Geometry check sheet. Reference: drawing and pictorial views, mm from the part's lowest x, y, z. Give positions to 0.01 mm unless a question says otherwise; leave off trailing zeros. Write each loop counter-clockwise with the first axis right and the second up, starting at its lowest first coordinate (ties: lowest second). Pieces come first, ordered by that corner, then holes. Notation, with made-up numbers: M 47.25,41.5 L 100.25,41.5 A28 cw 100.25,71.5 Z; hole C 2.25,29 d3. An arc over 180 degrees is marked long. Answer as a JSON object with one key per item and string values.
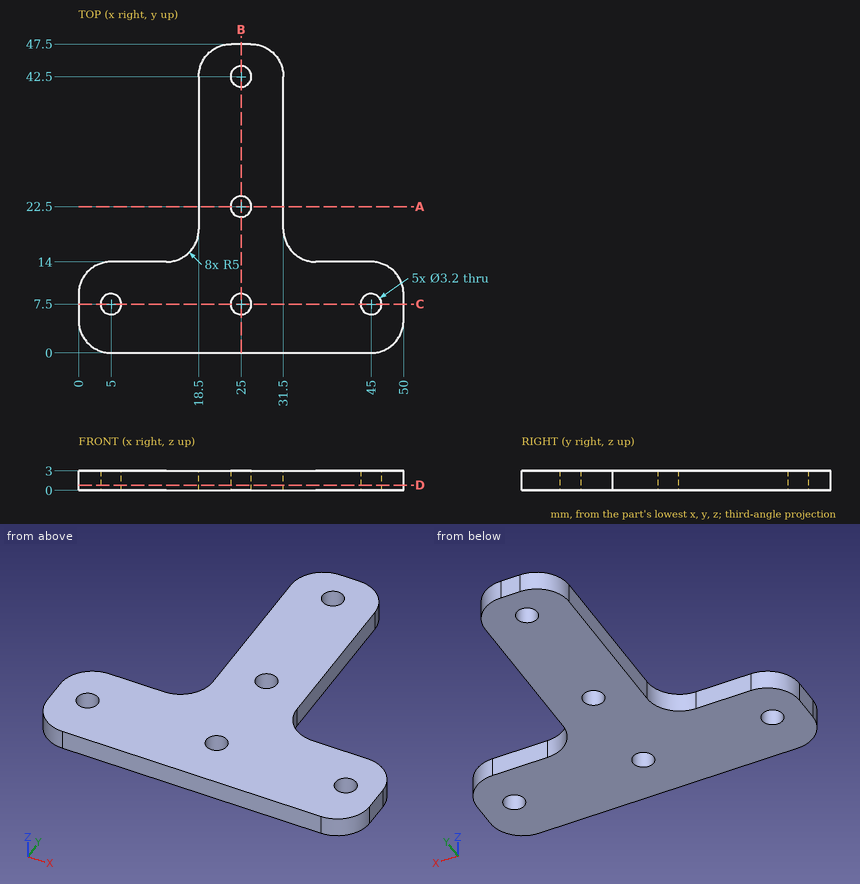
1) Section check C-C on y = 7.5. Record the boundary of the cut face in (x, z), and give its area (3 significant figures).
Completed:
{"outline": "M 0,0 L 3.4,0 L 3.4,3 L 0,3 Z; M 6.6,0 L 23.4,0 L 23.4,3 L 6.6,3 Z; M 26.6,0 L 43.4,0 L 43.4,3 L 26.6,3 Z; M 46.6,0 L 50,0 L 50,3 L 46.6,3 Z", "area": "121 mm2"}
2) Thickness scan on L1, parallel to Y at x = 25, z = 1.1; L2, parallel to Y at x = 12, z = 0.45; L3, parallel to X at y = 31.5, z = 0.45. Record the ranges inside material, lowest first.
Completed:
{"L1": "y = 0 to 5.9, 9.1 to 20.9, 24.1 to 40.9, 44.1 to 47.5", "L2": "y = 0 to 14", "L3": "x = 18.5 to 31.5"}
3) Section check B-B on x = 25. Record the boundary of the cut face in (y, z).
Completed:
{"outline": "M 0,0 L 5.9,0 L 5.9,3 L 0,3 Z; M 9.1,0 L 20.9,0 L 20.9,3 L 9.1,3 Z; M 24.1,0 L 40.9,0 L 40.9,3 L 24.1,3 Z; M 44.1,0 L 47.5,0 L 47.5,3 L 44.1,3 Z"}
4) Go/stop test with flat-tipped pins: pin 1 (0.9 mm diameter, centred on x = 8.5, z = 1.5, fed in from +Y); pin 2 (0.9 mm diameter, centred on y = 26, z = 1.5, fed in from +X); pin 3 (5 mm diameter, centred on x = 45, y = 7.5, fed in from -Z); pin 4 (3 mm diameter, centred on x = 5, y = 7.5, fed in from -Z) (1 decimal). Record where each tip stops, or that it passes through.
Completed:
{"pin 1": "stops at y = 14", "pin 2": "stops at x = 31.5", "pin 3": "stops at z = 0", "pin 4": "passes through"}
5) Section check D-D on z = 0.8. Record the boundary of the cut face in (x, y).
Completed:
{"outline": "M 0,5 A5 ccw 5,0 L 45,0 A5 ccw 50,5 L 50,9 A5 ccw 45,14 L 36.5,14 A5 cw 31.5,19 L 31.5,42.5 A5 ccw 26.5,47.5 L 23.5,47.5 A5 ccw 18.5,42.5 L 18.5,19 A5 cw 13.5,14 L 5,14 A5 ccw 0,9 Z; hole C 5,7.5 d3.2; hole C 25,7.5 d3.2; hole C 25,22.5 d3.2; hole C 25,42.5 d3.2; hole C 45,7.5 d3.2"}
6) Section check A-A on y = 22.5. Record the boundary of the cut face in (x, z), and give its area (3 significant figures).
Completed:
{"outline": "M 18.5,0 L 23.4,0 L 23.4,3 L 18.5,3 Z; M 26.6,0 L 31.5,0 L 31.5,3 L 26.6,3 Z", "area": "29.4 mm2"}
